The listing builds one solid part. Answer for the finished solid, in the listing's coordinates (mm). A direction names the side the tool comes from. Coordinates: 2 decimals unless noted, no trailing zeros. Write each loop counter-clockwise with the first axis right and the second up, starting at its lowest first coordinate (ties: lowest second). Pieces come first, ordered by that corner, then holes.
from build123d import *

# Parameters (mm, degrees)
F0_W     = 25.4
F0_H     = 44.45
F1_DEPTH = 57.15
F2_R     = 12.7
F3_DEPTH = 25.4
F4_W     = 12.7
F4_H     = 44.45
F5_DEPTH = 12.7


with BuildPart() as f1:
    # F0 (on Right) → F1 (new body)
    with BuildSketch(Plane.YZ):
        with Locations((12.7, 22.225)):
            Rectangle(F0_W, F0_H)
    extrude(amount=F1_DEPTH)

    # F2 (on face) → F3 (cut)
    with BuildSketch(Plane.XZ):
        with Locations((28.575, 25.4)):
            Circle(F2_R)
    extrude(amount=-F3_DEPTH, mode=Mode.SUBTRACT)

    # F4 (on face) → F5 (cut)
    with BuildSketch(Plane.XZ):
        with BuildLine():
            Line((44.45, 0), (44.45, 44.45))
            Line((44.45, 44.45), (19.05, 44.45))
            Line((19.05, 44.45), (23.3271277432, 36.9650264494))
            ThreePointArc((23.3271277432, 36.9650264494), (35.4540269057, 36.0756259222), (41.275, 25.4))
            ThreePointArc((41.275, 25.4), (39.8442616467, 19.5439141111), (35.8744107184, 15.0072812429))
            Line((35.8744107184, 15.0072812429), (44.45, 0))
        make_face()
        with Locations((50.8, 22.225)):
            Rectangle(F4_W, F4_H)
    extrude(amount=-F5_DEPTH, mode=Mode.SUBTRACT)


solid = f1.part
1. Section C-C on x = 37.5 is taken. Give the vertices of the cut face in (y, z), then the cut area to 3 significant figures.
Results found:
outline: (0, 0) - (25.4, 0) - (25.4, 16.36) - (12.7, 16.36) - (12.7, 12.16) - (0, 12.16) - close; (12.7, 34.44) - (25.4, 34.44) - (25.4, 44.45) - (12.7, 44.45) - close
area: 489 mm2
2. A tool of negligible diameter and unlimited length cuts with its end or side. For faces 1 (the flat face through (46, 12.7, 27)), 2 (the flat face through (22, 15, 44.45)), from which of +Z, -Z, +X, -X, +Y, -Y can it reach the whole face along a straight path? Write none if from no direction.
Results found:
face 1: +Z, +X, -Y
face 2: +Z, +X, -X, +Y, -Y
3. For a pull along Z with two mould halves and no side action, classify faces 3 (the cylindrical face through (18.5, 15.34, 17.67)), 4 (the flat face through (21.16, 6.26, 40.76)), 5 (the flat face through (28, 25.4, 12)) as pulls with the +Z half, pulls with the -Z half, needs draft (parallel to the pull), parting line crosses it, or undercut.
Results found:
face 3: undercut
face 4: pulls with the +Z half
face 5: needs draft
4. Section B-B on z = 25.4 is taken. Give the vertices of the cut face in (x, y) (3 decimals).
Results found:
outline: (0, 0) - (15.875, 0) - (15.875, 25.4) - (0, 25.4) - close; (41.275, 12.7) - (57.15, 12.7) - (57.15, 25.4) - (41.275, 25.4) - close
5. Section D-D on y = 8 is taken. Give the vertices of the cut face in (x, z) (3 decimals).
Results found:
outline: (0, 0) - (44.45, 0) - (35.874, 15.007) arc R12.7 cw (long way) to (23.327, 36.965) - (19.05, 44.45) - (0, 44.45) - close
6. Flat-ended cylindrical pins translate along their axes: P1, Ø5, axis at x = 26.5, y = 7, coming from the +Z side; P2, Ø5, axis at x = 29, y = 11.5, coming from the +Z side; P3, Ø2, axis at x = 32, y = 11.5, coming from the +Z side. Find the tip coordinate at first contact, or state that the pin passes through.
Results found:
P1: stops at z = 13.55
P2: stops at z = 44.45
P3: stops at z = 13.5
7. Find the intervals of material crossed by L1, parallel to X at y = 16.75, z = 25.4 (3 decimals); L2, parallel to Y at x = 46, z = 31.5; L3, parallel to Z at x = 24.5, y = 24, in increasing order.
Results found:
L1: x = 0 to 15.875, 41.275 to 57.15
L2: y = 12.7 to 25.4
L3: z = 0 to 13.37, 37.43 to 44.45
8. Section A-A on y = 22 is taken. Give the vertices of the cut face in (x, z) (3 decimals).
Results found:
outline: (0, 0) - (57.15, 0) - (57.15, 44.45) - (0, 44.45) - close; hole circle Ø25.4 at (28.575, 25.4)
